Design review of the part shown in the three views and the two pictorial views. Dimensions are in mm from the part's minimum x, y and z. Give positions to 0.01 mm unless a question says otherwise; leave off trailing zeros. Loops run counter-clockwise (first coordinate to the right, second up) from the corner with the lowest first, then second, coordinate; pieces in that order, holes last. Notation, with made-up numbers: (-10, 27.5) -> (40, 27.5) arc R23 ccw to (40, 58.5) -> close; hole circle Ø10 at (46, -27.5). An arc over 180 degrees is marked (long way). Answer as CSV lines item,"result". Start each with the question number.
Item 1: Add section C-C on z = 20.75. State the section outline as (x, y) points, plus the area to 3 significant figures.
Item 2: The part is to be moulded in two halves that separate along Y. For the marked faces 1, 2 and 3, say which applies: +Y half, -Y half, draft (parallel to the pull), parting line (faces both ways), or undercut.
Item 3: Add section A-A on y = 10.25. State the section outline as (x, z) points, plus the area to 3 significant figures.
Item 4: For L1, parallel to Y at x = 10.25, z = 24.25; L2, parallel to Y at x = 10.25, z = 8.25; L3, parallel to X at y = 13, z = 2, list the stretches that pass through material, from the lowest coordinate up. Write a range as from..to.
Item 5: Add section D-D on z = 10.5. State the section outline as (x, y) points, plus the area to 3 significant figures.
Item 6: Clearance check with flat-ended pins moving along their axes: P1, Ø1, axis at x = 14.5, z = 26.5, coming from the -Y side; P2, Ø5, axis at x = 5, z = 3.5, coming from the +Y side; P3, Ø4, axis at x = 11.5, y = 11.5, coming from the -Z side. State where each tip first meets the part, or that it passes through.
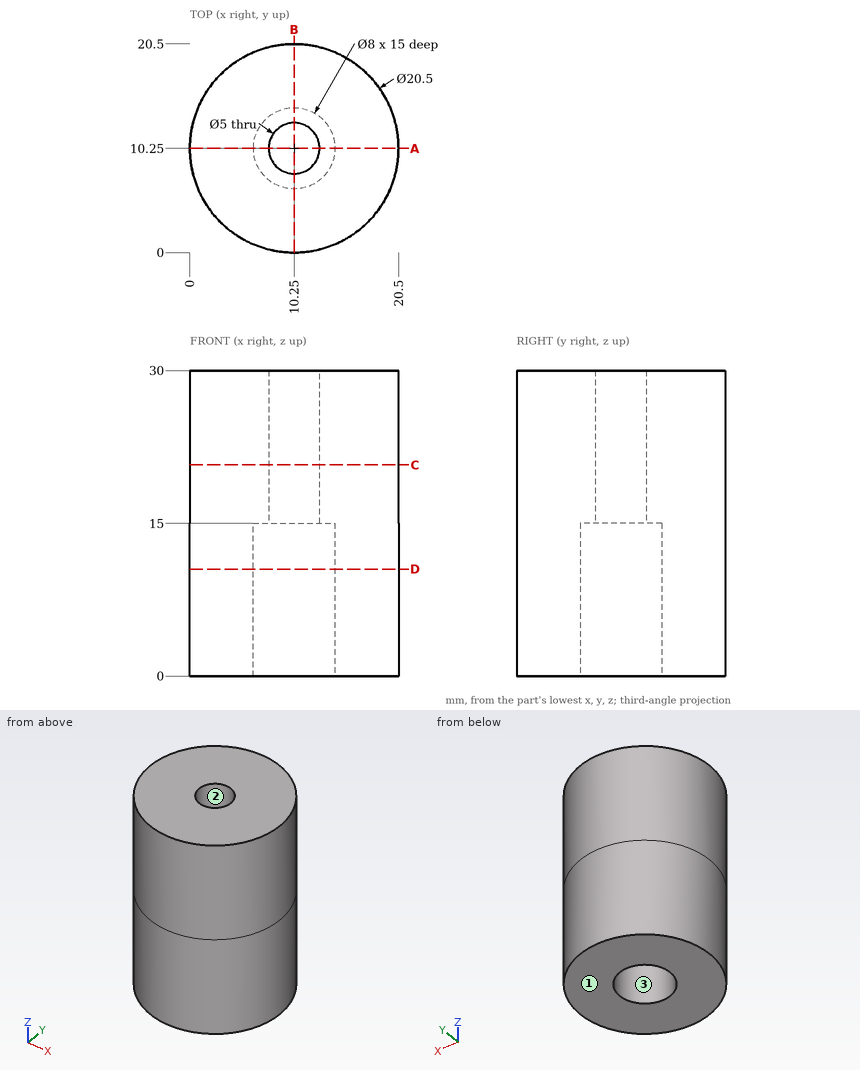
Computed values:
1,outline,"circle Ø20.5 at (10.25, 10.25); hole circle Ø5 at (10.25, 10.25)"
1,area,"310 mm²"
2,face 1,"draft"
2,face 2,"undercut"
2,face 3,"undercut"
3,outline,"(0, 0) -> (6.25, 0) -> (6.25, 15) -> (7.75, 15) -> (7.75, 30) -> (0, 30) -> close; (12.75, 15) -> (14.25, 15) -> (14.25, 0) -> (20.5, 0) -> (20.5, 30) -> (12.75, 30) -> close"
3,area,"420 mm²"
4,L1,"0..7.75, 12.75..20.5"
4,L2,"0..6.25, 14.25..20.5"
4,L3,"0.38..7.35, 13.15..20.12"
5,outline,"circle Ø20.5 at (10.25, 10.25); hole circle Ø8 at (10.25, 10.25)"
5,area,"280 mm²"
6,P1,"y = 0.71"
6,P2,"y = 20.12"
6,P3,"z = 15"
